Can you work these out from the model? Positions are in its coordinate system, mm. Face numbers are marked on the shaded views. Round coordinates to 2 decimals unless told otherwise and drop trailing zeros. Loops run counter-clockwise (first coordinate to the right, second up) from the corner with the lowest first, then second, coordinate; pieces in that order, holes last. Notation, with made-up numbers: (5, 13.5) - (28, 13.5) arc R14 ccw to (28, 18.5) - close; hole circle Ø4 at (82, 70). An arc over 180 degrees is marked (long way). Answer as CSV lines item,"result".
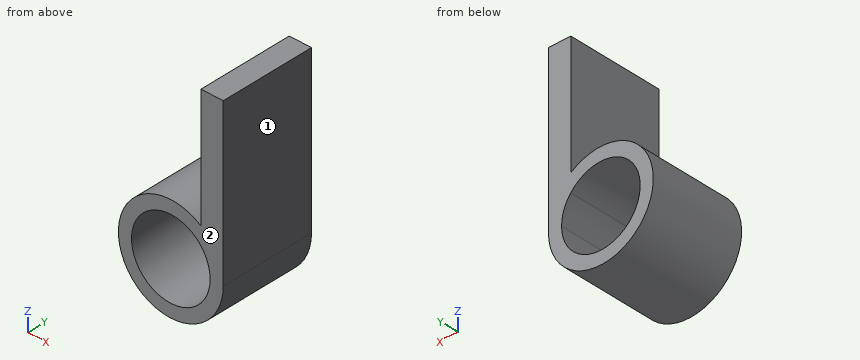
```python
from build123d import *

# Parameters (mm, degrees)
F1_DEPTH = 14.5


with BuildPart() as f1:
    # F0 (on Front) → F1 (new body)
    with BuildSketch(Plane.XZ):
        with BuildLine():
            ThreePointArc((8, 0), (7.099296, 3.687818), (4.6, 6.545227))
            ThreePointArc((4.6, 6.545227), (-7.099296, -3.687818), (8, 0))
        make_face()
        with BuildLine():
            ThreePointArc((4.6, 3.852272), (5.639149, 2.04939), (6, 0))
            ThreePointArc((6, 0), (-5.639149, -2.04939), (4.6, 3.852272))
        make_face(mode=Mode.SUBTRACT)
        with BuildLine():
            Line((4.6, 25), (4.6, 6.545227))
            ThreePointArc((4.6, 6.545227), (7.099296, 3.687818), (8, 0))
            Line((8, 0), (8, 25))
            Line((8, 25), (4.6, 25))
        make_face()
    extrude(amount=F1_DEPTH)


solid = f1.part
```
Q1. We'd pull the mould along X, two halves only. Please class the marked faces 1 and 2: pulls with the +X half, pulls with the -X half, needs draft (parallel to the pull), parting line crosses it, or undercut.
Checks:
face 1,"pulls with the +X half"
face 2,"needs draft"
Q2. If I drill on line 1 along Z through (x, y) = (0, -6.75); line 2 along X through (y, z) = (-6.5, 8.5); line 3 along Z through (x, y) = (-1.75, -9.75), over which ranges is the centre line in solid material (lowest first)? Write a range as [from, to].
Checks:
line 1,"[-8, -6], [6, 8]"
line 2,"[4.6, 8]"
line 3,"[-7.81, -5.74], [5.74, 7.81]"
Q3. Imagine slicing it at D-D (x = 3.75). Write out the boundary of the cut face in (y, z).
Checks:
outline,"(-14.5, -7.07) - (0, -7.07) - (0, -4.68) - (-14.5, -4.68) - close; (-14.5, 4.68) - (0, 4.68) - (0, 7.07) - (-14.5, 7.07) - close"
Q4. Imagine slicing it at C-C (z = 10.5). Write out the boundary of the cut face in (x, y), then the cut area to 3 significant figures.
Checks:
outline,"(4.6, -14.5) - (8, -14.5) - (8, 0) - (4.6, 0) - close"
area,"49.3 mm²"
Q5. I'm going to push flat-ended pins straight in: pin 1 Ø4 at (x, y) = (-1.5, -5) entering from +Z; pin 2 Ø9.5 at (x, z) = (0, 0) entering from -Y; pin 3 Ø1.5 at (x, y) = (-2.5, -3.5) entering from +Z; pin 4 Ø4.5 at (y, z) = (-3.5, 20.5) entering from -X. Where does each tip first touch, or does it pass through?
Checks:
pin 1,"z = 8"
pin 2,"through"
pin 3,"z = 7.81"
pin 4,"x = 4.6"
Q6. Imagine slicing it at A-A (x = 0). Write out the boundary of the cut face in (y, z).
Checks:
outline,"(-14.5, -8) - (0, -8) - (0, -6) - (-14.5, -6) - close; (-14.5, 6) - (0, 6) - (0, 8) - (-14.5, 8) - close"
Q7. Imagine slicing it at B-B (y = -4.5). Write out the boundary of the cut face in (x, z).
Checks:
outline,"(4.6, 6.55) arc R8 ccw (long way) to (8, 0) - (8, 25) - (4.6, 25) - close; hole (4.6, 3.85) arc R6 ccw (long way) to (6, 0) arc R6 ccw to start"
